Part model, mm, in its own coordinate system. Face numbers are marked on the shaded views. A direction names the side the tool comes from. Give positions to 0.01 mm unless a question says otherwise; leave off trailing zeros. Write each loop counter-clockwise with the first axis right and the second up, starting at its lowest first coordinate (ties: lowest second). Pieces come first, ordered by that corner, then holes. Notation, with made-up numbers: M 74,-11.75 L 111,-11.75 A33 cw 111,16.25 Z; hole C 75.25,66 d8. An arc over 180 degrees is marked long. Write item = value, one per line. Start each with the question number.
Autodesk Inventor part; units mm, degrees
ref_plane "YZ Plane" through (0, 0, 0) normal (1, 0, 0) x (0, 1, 0)
ref_plane "XZ Plane" through (0, 0, 0) normal (0, 1, 0) x (-1, 0, 0)
ref_plane "XY Plane" through (0, 0, 0) normal (0, 0, 1) x (1, 0, 0)
sketch "Sketch1" plane through (0, 0, 0) normal (0, 1, 0) x (-1, 0, 0)
  circle A0 centre (0, 0) radius 15
  circle A1 centre (0, 0) radius 10
  line L0 (0, 0) -> (-15, 0)
  line L1 (-15, 0) -> (-7.5, 12.9904)
  line L2 (-7.5, 12.9904) -> (0, 0)
  line L3 (-7.5, 12.9904) -> (7.5, 12.9904)
  line L4 (7.5, 12.9904) -> (15, 0)
  line L5 (15, 0) -> (7.5, -12.9904)
  line L6 (7.5, -12.9904) -> (-7.5, -12.9904)
  line L7 (-7.5, -12.9904) -> (-15, 0)
  line L8 (0, 0) -> (7.5, 12.9904)
  line L9 (0, 0) -> (15, 0)
  line L10 (0, 0) -> (7.5, -12.9904)
  line L11 (0, 0) -> (-7.5, -12.9904)
extrude "Extrusion3" add sketch "Sketch1" along normal blind 5 contours L7 L0 A1 L11 | L11 A1 L0
sketch "Sketch5" plane through (7.5, 0, -12.9904) normal (0.866, 0, -0.5) x (-0.5, 0, -0.866)
  line L0 (-15, 0) -> (0, 0)
  line L1 (0, 0) -> (0, 5)
  line L2 (-15, 5) -> (0, 5)
  line L3 (-15, 0) -> (-15, 5)
  line L4 (0, 0) -> (-15, 5)
  line L5 (-15, 0) -> (0, 5)
  line L6 (-7.5, 2.5) -> (-7.5, 5)
  line L7 (-7.5, 5) -> (-10, 5)
  line L8 (-10, 5) -> (-7.5, 2.5)
  line L9 (-7.5, 2.5) -> (-5, 0)
  line L10 (-10, 5) -> (-8.75, 5)
  line L11 (-8.75, 5) -> (-3.75, 0)
  line L12 (-3.75, 0) -> (-6.25, 0)
  line L13 (-6.25, 0) -> (-11.25, 5)
  line L14 (-10, 5) -> (-11.25, 5)
  dimension "d18" = 2.5
  dimension "d19" = 2.5
extrude "Extrusion4" add sketch "Sketch5" along normal blind 5 contours L13 L5 L9 L0 | L13 L4 L5 | L9 L4 L11 L0 | L2 L8 L4 L13 | L5 L11 L4 | L6 L11 L5 | L8 L2 L11 L6
sketch "Sketch6" plane through (11.875, 5, -5.4127) normal (-0.3536, 0.7071, -0.6124) x (0.866, 0, -0.5)
  line L0 (0, 0) -> (0, 7.0711)
  line L1 (0, 0) -> (5, 0)
  line L2 (5, 7.0711) -> (5, 0)
  line L3 (0, 7.0711) -> (5, 7.0711)
  line L4 (0, 0) -> (5, 7.0711)
  line L5 (5, 0) -> (0, 7.0711)
  line L6 (2.5, 3.5355) -> (2.5, 2.7855)
  line L7 (2.5, 2.7855) -> (3.5, 2.7855)
  circle A0 centre (3.5, 2.7855) radius 0.4
  point P0 (3.2526, 2.4712)
  point P1 (3.1212, 2.657)
  dimension "d22" = 0.75
  dimension "d26" = 1
  dimension "d27" = 0.8
extrude "Extrusion5" cut sketch "Sketch6" against normal blind 5 contours L5 A0 picked at (3.3911, 2.7263)
pattern_circular "Circular Pattern1" count 6 over 360 about axis through (0, 0, 0) along (0, 1, 0) of "Extrusion3", "Extrusion4", "Extrusion5"
properties part number "hub"
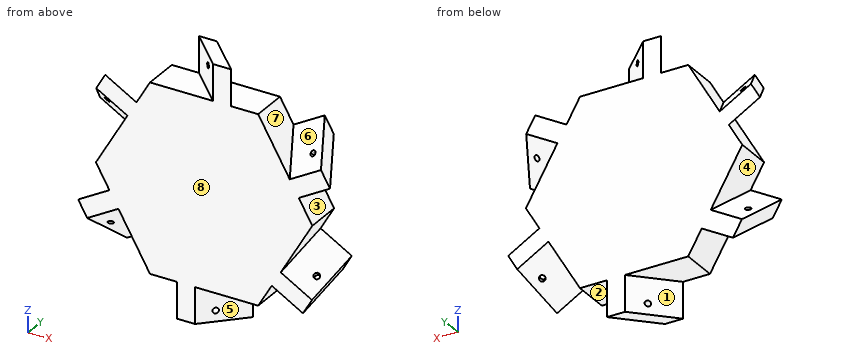
Q1. Drop flat-ended pins along their axis: P1, Ø2, axis at y = 2.5, z = 4, coming from the +X side; P2, Ø2.5, axis at x = 5, y = 3, coming from the +Z side; P3, Ø1.5, axis at y = 1.5, z = -3, coming from the -X side. Give the stop position or say it passes through.
Q2. Slice it at A-A (z = -10.5). Give the cut face in (x, y).
Q3. Tool access for the marked faces 1, 2, 3 and 4: list every direction of +Z, -Z, +X, -X, +Y, -Y with a clear straight run to the whole face (end or side of a thin tool).
Q4. Probe line 1 along X through (y, z) = (1.9, 8); line 2 along Z through (x, y) = (5, 3.65); line 3 along Z through (x, y) = (-2, 3.45). List the from-to ranges inside material, lowest first.
Q5. Slice it at D-D (x = -10). Give the cut face in (y, z).
Q6. Slice it at B-B (x = 6). Give the cut face in (y, z).
Q7. Slice it at C-C (z = 14). Give the cut face in (x, y).
Q8. Two-plate mould, pull along X, no slides. Class the marked faces 5, 6, 7 and 8: +X half, -X half, draft (parallel to the pull), parting line (faces both ways), or undercut.
Working result:
q1.P1 = 13.27
q1.P2 = 12.99
q1.P3 = -13.7
q2.outline = M -14.71,2.99 L -10.69,5 L -14.71,5 Z; M -8.94,0 L 8.94,0 L 8.94,5 L -8.94,5 Z; M 10.69,0 L 14.71,0 L 14.71,2.01 Z
q3.face_1 = -Z, -X, +Y
q3.face_2 = -Z, +X, -Y
q3.face_3 = +X, +Y
q3.face_4 = -X, +Y
q4.line_1 = -15.16 to -14.88, -14.04 to 10.38, 12.56 to 16.15
q4.line_2 = -12.99 to 12.99
q4.line_3 = -12.99 to 17.99
q5.outline = M 0,-8.66 L 3.75,-8.66 L 5,-10.1 L 5,8.66 L 1.25,8.66 L 0,10.1 Z
q6.outline = M 0,-12.99 L 5,-12.99 L 5,12.99 L 0,12.99 Z
q7.outline = M -3.75,5 L 1.25,0 L 3.75,0 L -1.25,5 Z
q8.face_5 = +X half
q8.face_6 = undercut
q8.face_7 = undercut
q8.face_8 = draft
